Geometry: final body of the model. Coordinates: model frame, mm. A direction names the side the tool comes from. Coordinates: 2 decimals unless noted, no trailing zeros. Write each loop counter-clockwise with the first axis right and the second up, starting at its lowest first coordinate (ties: lowest second). Pieces come first, ordered by that corner, then holes. Notation, with made-up numbers: (9.5, 34) -> (47.5, 34) arc R13 cw to (47.5, 42) -> close; hole circle Ø9 at (72.25, 54). An arc over 180 degrees is marked (long way). One line per item, written item: value.
```python
from build123d import *

# Parameters (mm, degrees)
SKETCH1_R                  = 31
BASE_EXTRUDE_DEPTH         = 12.5
SKETCH4_R                  = 7.125
F_4_STK_14_25_HULLER_DEPTH = 25


with BuildPart() as part:
    # Sketch1 → Base-Extrude (new body, symmetric)
    with BuildSketch(Plane.XY):
        with BuildLine():
            Line((34, 46), (21.540659229, 46))
            ThreePointArc((21.540659229, 46), (19.71491737, 46.168079197), (17.950549357, 46.666666667))
            ThreePointArc((17.950549357, 46.666666667), (0, 50), (-17.950549357, 46.666666667))
            ThreePointArc((-17.950549357, 46.666666667), (-19.71491737, 46.168079197), (-21.540659229, 46))
            Line((-21.540659229, 46), (-34, 46))
            ThreePointArc((-34, 46), (-42.485281374, 42.485281374), (-46, 34))
            Line((-46, 34), (-46, 17))
            ThreePointArc((-46, 17), (-47.658359214, 14.316718427), (-50.8, 14.6))
            Line((-50.8, 14.6), (-53.2, 16.4))
            ThreePointArc((-53.2, 16.4), (-56.341640786, 16.683281573), (-58, 14))
            Line((-58, 14), (-58, -14))
            ThreePointArc((-58, -14), (-56.341640786, -16.683281573), (-53.2, -16.4))
            Line((-53.2, -16.4), (-50.8, -14.6))
            ThreePointArc((-50.8, -14.6), (-47.658359214, -14.316718427), (-46, -17))
            Line((-46, -17), (-46, -34))
            ThreePointArc((-46, -34), (-42.485281374, -42.485281374), (-34, -46))
            Line((-34, -46), (-21.540659229, -46))
            ThreePointArc((-21.540659229, -46), (-19.71491737, -46.168079197), (-17.950549357, -46.666666667))
            ThreePointArc((-17.950549357, -46.666666667), (0, -50), (17.950549357, -46.666666667))
            ThreePointArc((17.950549357, -46.666666667), (19.71491737, -46.168079197), (21.540659229, -46))
            Line((21.540659229, -46), (34, -46))
            ThreePointArc((34, -46), (42.485281374, -42.485281374), (46, -34))
            Line((46, -34), (46, -17))
            ThreePointArc((46, -17), (47.658359214, -14.316718427), (50.8, -14.6))
            Line((50.8, -14.6), (53.2, -16.4))
            ThreePointArc((53.2, -16.4), (56.341640786, -16.683281573), (58, -14))
            Line((58, -14), (58, 14))
            ThreePointArc((58, 14), (56.341640786, 16.683281573), (53.2, 16.4))
            Line((53.2, 16.4), (50.8, 14.6))
            ThreePointArc((50.8, 14.6), (47.658359214, 14.316718427), (46, 17))
            Line((46, 17), (46, 34))
            ThreePointArc((46, 34), (42.485281374, 42.485281374), (34, 46))
        make_face()
        Circle(SKETCH1_R, mode=Mode.SUBTRACT)
    extrude(amount=BASE_EXTRUDE_DEPTH, both=True)

    # Sketch2 → Uddrejning (revolve, cut)
    with BuildSketch(Plane(origin=(0, 0, 0), x_dir=(0, 0, -1), z_dir=(1, 0, 0))):
        Polygon((11.5, 38.5), (4.5, 38.5), (4.5, 35), (-12.5, 35), (-12.5, 0), (12.5, 0), (12.5, 70), (11.5, 70), align=None)
    revolve(axis=Axis((0, 0, 0), (0, 0, -1)), mode=Mode.SUBTRACT)

    # Sketch4 → 4 stk ø14.25 huller (cut, through all)
    with BuildSketch(Plane.XY.offset(-11.5)):
        with Locations((33.587572106, 33.587572106)):
            Circle(SKETCH4_R)
        with Locations((33.587572106, -33.587572106)):
            Circle(SKETCH4_R)
        with Locations((-33.587572106, -33.587572106)):
            Circle(SKETCH4_R)
        with Locations((-33.587572106, 33.587572106)):
            Circle(SKETCH4_R)
    extrude(amount=F_4_STK_14_25_HULLER_DEPTH, mode=Mode.SUBTRACT)


solid = part.part
```
(1) First-contact query: pin 1 (3.5 mm diameter, centred on x = 26, z = -1.5, fed in from -Y); pin 2 (3 mm diameter, centred on y = 32.5, z = -2.5, fed in from -X); pin 3 (5 mm diameter, centred on y = 24.5, z = -4.5, fed in from +X). Flat tips, straight axial feed; report the tip coordinate or a pass-through.
Responses:
pin 1: stops at y = -46
pin 2: stops at x = -46
pin 3: stops at x = 46
(2) Reachability of faces 1 (the flat face through (52, -15.5, 0.7)), 2 (the flat face through (28, -46, 1)), 3 (the flat face through (28, 46, 1)), 4 (the cylindrical face through (-47.617, 14.338, 0.668)), 5 (the flat face through (-46, 26, 1)) from +Z, -Z, +X, -X, +Y, -Y: full face, straight path, thin tool, end or side. Return the list, or none.
Responses:
face 1: +Z, -Z, -Y
face 2: +Z, -Z, +X, -Y
face 3: +Z, -Z, +X, +Y
face 4: +Z, -Z, +Y
face 5: +Z, -Z, -X, +Y
(3) Section B-B (y = 0). Return the cut outline in (x, z), then the cut area to 4 significant figures.
Responses:
outline: (-58, -11.5) -> (-38.5, -11.5) -> (-38.5, -4.5) -> (-35, -4.5) -> (-35, 12.5) -> (-58, 12.5) -> close; (35, -4.5) -> (38.5, -4.5) -> (38.5, -11.5) -> (58, -11.5) -> (58, 12.5) -> (35, 12.5) -> close
area: 1,055 mm2
(4) Line query: line 1 (X direction, y = 0, z = 2.5); line 2 (Y direction, x = 32, z = 6); line 3 (Y direction, x = -40, z = -2.75). Output: solid intervals per line, ascending. Write a range as [from, to].
Responses:
line 1: x = [-58, -35], [35, 58]
line 2: y = [-46, -40.53], [-26.64, -14.18], [14.18, 26.64], [40.53, 46]
line 3: y = [-44.39, -36.69], [-30.48, 30.48], [36.69, 44.39]
(5) Section C-C (x = 32). Return the cut outline in (y, z).
Responses:
outline: (-46, -11.5) -> (-40.53, -11.5) -> (-40.53, 12.5) -> (-46, 12.5) -> close; (-26.64, -11.5) -> (-21.41, -11.5) -> (-21.41, -4.5) -> (-14.18, -4.5) -> (-14.18, 12.5) -> (-26.64, 12.5) -> close; (14.18, -4.5) -> (21.41, -4.5) -> (21.41, -11.5) -> (26.64, -11.5) -> (26.64, 12.5) -> (14.18, 12.5) -> close; (40.53, -11.5) -> (46, -11.5) -> (46, 12.5) -> (40.53, 12.5) -> close
(6) Pull-direction query (Y, two-part tool) for faces 6 (the flat face through (-46, -25, 1)), 7 (the cylindrical face through (-23.43, -30.55, -7.95)), 8 (the cylindrical face through (-26.79, -31.45, 0.33)), 9 (the cylindrical face through (42.58, 42.39, 0.67)); classes: released by +Y, released by -Y, zero draft, split by the parting line, or undercut.
Responses:
face 6: zero draft
face 7: undercut
face 8: undercut
face 9: released by +Y
(7) Section A-A (x = 0). Return the cut outline in (y, z), then the cut area to 3 significant figures.
Responses:
outline: (-50, -11.5) -> (-38.5, -11.5) -> (-38.5, -4.5) -> (-35, -4.5) -> (-35, 12.5) -> (-50, 12.5) -> close; (35, -4.5) -> (38.5, -4.5) -> (38.5, -11.5) -> (50, -11.5) -> (50, 12.5) -> (35, 12.5) -> close
area: 671 mm2
(8) Section D-D (z = 4.5). State how many separate pieces and enclosed holes the cut face has, then the cut area to 3 significant figures.
Responses:
separate pieces: 1
enclosed holes: 5
area: 4,810 mm2
